Autodesk Inventor part; units mm, degrees
ref_plane "YZ Plane" through (0, 0, 0) normal (1, 0, 0) x (0, 1, 0)
ref_plane "XZ Plane" through (0, 0, 0) normal (0, 1, 0) x (-1, 0, 0)
ref_plane "XY Plane" through (0, 0, 0) normal (0, 0, 1) x (1, 0, 0)
sketch "Sketch1" plane through (0, 0, 0) normal (0, 0, 1) x (1, 0, 0)
  circle A0 centre (0, 0) radius 1.59
  line L0 (-12.5, 15) -> (7.5, 15)
  line L1 (7.5, 15) -> (7.5, -15)
  line L2 (7.5, -15) -> (-12.5, -15)
  line L3 (-12.5, -15) -> (-12.5, 15)
  circle A1 centre (-7.5, 11.25) radius 1.59
  line L4 (-3, 5) -> (3, 5) construction
  line L5 (-3, 3.4125) -> (3, 3.4125)
  line L6 (3, 6.5875) -> (-3, 6.5875)
  arc A2 (-3, 6.5875) -> (-3, 3.4125) centre (-3, 5) ccw
  arc A3 (3, 3.4125) -> (3, 6.5875) centre (3, 5) ccw
  line L7 (-3, -5) -> (3, -5) construction
  line L8 (-3, -6.5875) -> (3, -6.5875)
  line L9 (3, -3.4125) -> (-3, -3.4125)
  arc A4 (-3, -3.4125) -> (-3, -6.5875) centre (-3, -5) ccw
  arc A5 (3, -6.5875) -> (3, -3.4125) centre (3, -5) ccw
  line L10 (-12.5, -3.4125) -> (7.5, -3.4125)
  point P0 (7.5, 0)
  point P1 (0, 5)
  point P2 (0, -5)
  point P3 (0, 0)
  dimension "d2" = 3.18
  dimension "d31" = 20
  dimension "d32" = 30
  dimension "d33" = 10
  dimension "d35" = 5
  dimension "d39" = 3.175
  dimension "d41" = 6
  dimension "d42" = 9.175
  dimension "d44" = 7.5
  dimension "d45" = 15
  dimension "d46" = 11.25
extrude "Extrusion1" add sketch "Sketch1" along normal blind 3.175 contours L0 L1 L10 L9 L3
fillet "Fillet1" radius 2 4 edges at (-12.5, 15, 1.5875) (7.5, 15, 1.5875) (7.5, -3.4125, 1.5875) (-12.5, -3.4125, 1.5875)
equation "\"d12\" = THICKA"
equation "\"THICKA\" = 3.175"
equation "\"THICKB\" = 6.731"
equation "\"THICKC\" = 12.7"
equation "\"MAGDIA\" = 9.5"
equation "\"BALLDIA\" = 12"
equation "\"THICKPLY\" = 5"
properties part number "Carriage_Joint_Beltflap"
Here's how the part is built. I have some questions about the finished solid (model axes, mm). A direction names the side the tool comes from. Coordinates: 2 decimals unless noted, no trailing zeros. Loops run counter-clockwise (first coordinate to the right, second up) from the corner with the lowest first, then second, coordinate; pieces in that order, holes last.
1. For faces 4 (the flat face through (-2, -3.412, 2)), 5 (the cylindrical face through (4.587, 5.035, 1.565)), which set-ups out of +Z, -Z, +X, -X, +Y, -Y let a thin tool reach every point of the face, with its end or its side?
2. If we mould it in two halves opening along X, with no side actions, what happens to faces 1 (the flat face through (-5, 6, 3.175)), 2 (the cylindrical face through (-11.93, -2.81, 1.61)), 3 (the cylindrical face through (-0.345, 1.552, 1.565))? For each: pulls with the +X half, pulls with the -X half, needs draft (parallel to the pull), parting line crosses it, or undercut.
3. Imagine slicing it at A-A, the plane x = -7.5. Please give me the cut outline in (y, z) (1 decimal).
4. Imagine slicing it at B-B, the plane y = 11.25. Please give me the cut outline in (x, z) (3 decimals).
5. Imagine slicing it at C-C, the plane x = 0. Please give me the cut outline in (y, z) (1 decimal).
6. I need wall thicknesses on L1, parallel to Y at x = 0, z = 1.2; L2, parallel to Y at x = -7.5, z = 2.45; L3, parallel to Y at x = -1, z = 2.9. Which ranges of each line are inside material? Lowest first, please.
7. Imagine slicing it at D-D, the plane z = 0.9. Count the separate pieces of the cut face and the enclosed holes in it, and give its area (3 significant figures).
Taken from the geometry:
1. face 4: +Z, -Z, +X, -X, -Y
1. face 5: +Z, -Z
2. face 1: needs draft
2. face 2: pulls with the -X half
2. face 3: undercut
3. outline: (-3.4, 0) - (9.7, 0) - (9.7, 3.2) - (-3.4, 3.2) - close; (12.8, 0) - (15, 0) - (15, 3.2) - (12.8, 3.2) - close
4. outline: (-12.5, 0) - (-9.09, 0) - (-9.09, 3.175) - (-12.5, 3.175) - close; (-5.91, 0) - (7.5, 0) - (7.5, 3.175) - (-5.91, 3.175) - close
5. outline: (-3.4, 0) - (-1.6, 0) - (-1.6, 3.2) - (-3.4, 3.2) - close; (1.6, 0) - (3.4, 0) - (3.4, 3.2) - (1.6, 3.2) - close; (6.6, 0) - (15, 0) - (15, 3.2) - (6.6, 3.2) - close
6. L1: y = -3.41 to -1.59, 1.59 to 3.41, 6.59 to 15
6. L2: y = -3.41 to 9.66, 12.84 to 15
6. L3: y = -3.41 to -1.24, 1.24 to 3.41, 6.59 to 15
7. separate pieces: 1
7. enclosed holes: 3
7. area: 322 mm2
